Geometry: see drawing. Coordinates: mm, zero at the bounding-box minimum. A direction names the side the tool comes from. Give positions to 0.01 mm unless a question says otherwise; leave off trailing zeros. Write each loop counter-clockwise with the first axis right and the second up, starting at its lowest first coordinate (ties: lowest second). Pieces come first, ordered by that corner, then holes. Notation, with made-up numbers: (-7.75, 47) -> (22.25, 47) arc R25 cw to (22.25, 62) -> close; hole circle Ø5 at (71.25, 43.5). An arc over 180 degrees is marked (long way). Use one line per item in the form item = value. Start each with the question number.
(1) Cut plane D-D, the plane z = 2.75. Output: boundary loops of the cut face in (x, y).
(2) Cut plane C-C, the plane y = 15. Output: boundary loops of the cut face in (x, z), and give its area (3 significant figures).
(3) Cut plane A-A, the plane x = 5. Output: boundary loops of the cut face in (y, z).
(4) First-contact query: P1, Ø3, axis at y = 15.5, z = 3, coming from the -X side; P2, Ø5.5, axis at x = 15, z = 5, coming from the -Y side; P3, Ø1, axis at x = 23.5, z = 5, coming from the +Y side. Flat tips, straight axial feed; report the tip coordinate or a pass-through.
(5) Material intervals for line 1 along Z through (x, y) = (5, 1.5); line 2 along Y through (x, z) = (24.75, 2.5); line 3 along X through (y, z) = (14.75, 6.75), sorted ascending. Write a range as from..to.
(6) Cut plane B-B, the plane z = 5. Output: boundary loops of the cut face in (x, y), and give its area (3 significant figures).
(7) Set-up query: the marked faces 1 and 2. Return all of +Z, -Z, +X, -X, +Y, -Y with unobstructed straight access to the full face (end or side cutting, diameter ignored); none if empty.
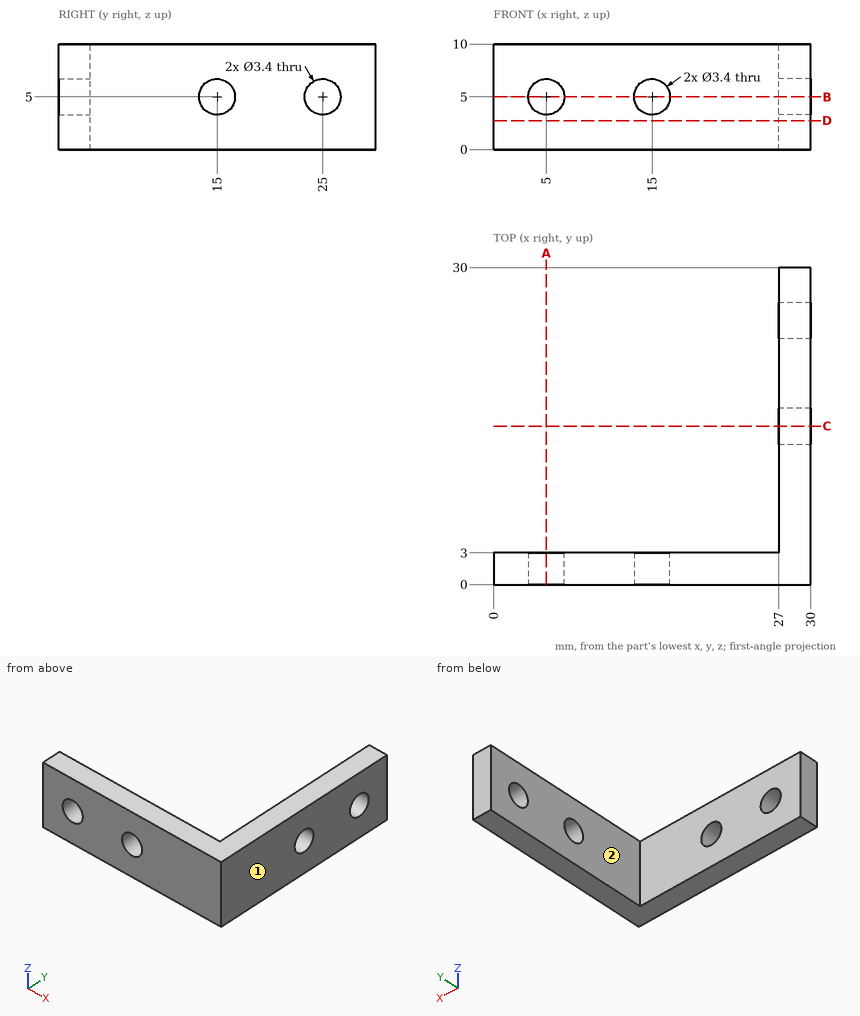
Geometry says:
q1.outline = (0, 0) -> (30, 0) -> (30, 30) -> (27, 30) -> (27, 3) -> (0, 3) -> close
q2.outline = (27, 0) -> (30, 0) -> (30, 3.3) -> (27, 3.3) -> close; (27, 6.7) -> (30, 6.7) -> (30, 10) -> (27, 10) -> close
q2.area = 19.8 mm^2
q3.outline = (0, 0) -> (3, 0) -> (3, 3.3) -> (0, 3.3) -> close; (0, 6.7) -> (3, 6.7) -> (3, 10) -> (0, 10) -> close
q4.P1 = 27
q4.P2 = 0
q4.P3 = 3
q5.line_1 = 0..3.3, 6.7..10
q5.line_2 = 0..3
q5.line_3 = 27..30
q6.outline = (0, 0) -> (3.3, 0) -> (3.3, 3) -> (0, 3) -> close; (6.7, 0) -> (13.3, 0) -> (13.3, 3) -> (6.7, 3) -> close; (16.7, 0) -> (30, 0) -> (30, 13.3) -> (27, 13.3) -> (27, 3) -> (16.7, 3) -> close; (27, 16.7) -> (30, 16.7) -> (30, 23.3) -> (27, 23.3) -> close; (27, 26.7) -> (30, 26.7) -> (30, 30) -> (27, 30) -> close
q6.area = 130 mm^2
q7.face_1 = +Z, -Z, +X, +Y, -Y
q7.face_2 = +Z, -Z, -X, +Y
